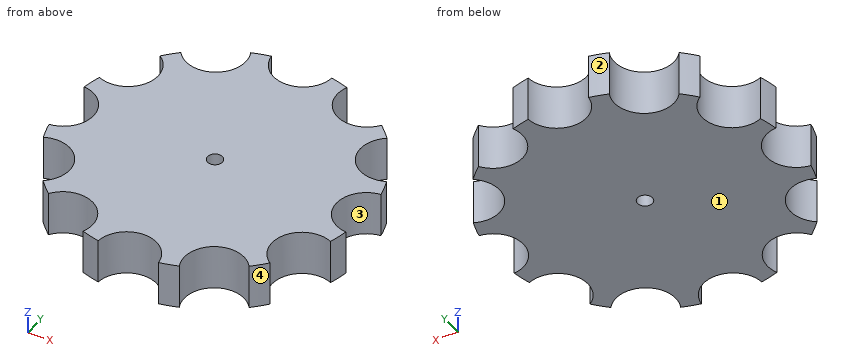
```python
from build123d import *

# Parameters (mm, degrees)
BOSS_EXTRUDE3_DEPTH = 15
SKETCH3_R           = 2.5
CUT_EXTRUDE2_DEPTH  = 15


with BuildPart() as part:
    # Sketch1 → Boss-Extrude3 (new body)
    with BuildSketch(Plane.XY):
        with BuildLine():
            ThreePointArc((48.999319531, 9.953224878), (48.296291314, 12.940952255), (47.411267921, 15.879914172))
            ThreePointArc((47.411267921, 15.879914172), (34.638070137, 19.998299118), (37.458043043, 33.119405359))
            ThreePointArc((37.458043043, 33.119405359), (35.355339059, 35.355339059), (33.119405359, 37.458043043))
            ThreePointArc((33.119405359, 37.458043043), (19.998299118, 34.638070137), (15.879914172, 47.411267921))
            ThreePointArc((15.879914172, 47.411267921), (12.940952255, 48.296291314), (9.953224878, 48.999319531))
            ThreePointArc((9.953224878, 48.999319531), (0, 39.996598235), (-9.953224878, 48.999319531))
            ThreePointArc((-9.953224878, 48.999319531), (-12.940952255, 48.296291314), (-15.879914172, 47.411267921))
            ThreePointArc((-15.879914172, 47.411267921), (-19.998299118, 34.638070137), (-33.119405359, 37.458043043))
            ThreePointArc((-33.119405359, 37.458043043), (-35.355339059, 35.355339059), (-37.458043043, 33.119405359))
            ThreePointArc((-37.458043043, 33.119405359), (-34.638070137, 19.998299118), (-47.411267921, 15.879914172))
            ThreePointArc((-47.411267921, 15.879914172), (-48.296291314, 12.940952255), (-48.999319531, 9.953224878))
            ThreePointArc((-48.999319531, 9.953224878), (-39.996598235, 0), (-48.999319531, -9.953224878))
            ThreePointArc((-48.999319531, -9.953224878), (-48.296291314, -12.940952255), (-47.411267921, -15.879914172))
            ThreePointArc((-47.411267921, -15.879914172), (-34.638070137, -19.998299118), (-37.458043043, -33.119405359))
            ThreePointArc((-37.458043043, -33.119405359), (-35.355339059, -35.355339059), (-33.119405359, -37.458043043))
            ThreePointArc((-33.119405359, -37.458043043), (-19.998299118, -34.638070137), (-15.879914172, -47.411267921))
            ThreePointArc((-15.879914172, -47.411267921), (-12.940952255, -48.296291314), (-9.953224878, -48.999319531))
            ThreePointArc((-9.953224878, -48.999319531), (0, -39.996598235), (9.953224878, -48.999319531))
            ThreePointArc((9.953224878, -48.999319531), (12.940952255, -48.296291314), (15.879914172, -47.411267921))
            ThreePointArc((15.879914172, -47.411267921), (19.998299118, -34.638070137), (33.119405359, -37.458043043))
            ThreePointArc((33.119405359, -37.458043043), (35.355339059, -35.355339059), (37.458043043, -33.119405359))
            ThreePointArc((37.458043043, -33.119405359), (34.638070137, -19.998299118), (47.411267921, -15.879914172))
            ThreePointArc((47.411267921, -15.879914172), (48.296291314, -12.940952255), (48.999319531, -9.953224878))
            ThreePointArc((48.999319531, -9.953224878), (39.996598235, 0), (48.999319531, 9.953224878))
        make_face()
    extrude(amount=BOSS_EXTRUDE3_DEPTH)

    # Sketch3 → Cut-Extrude2 (cut)
    with BuildSketch(Plane(origin=(0, 0, 0), x_dir=(-1, 0, 0), z_dir=(0, 0, -1))):
        Circle(SKETCH3_R)
    extrude(amount=-CUT_EXTRUDE2_DEPTH, mode=Mode.SUBTRACT)


solid = part.part
```
Input: part model. Units: mm. Frame: model coordinates. Face numbers are marked on the shaded views. Coordinates: 2 decimals unless noted, no trailing zeros. Write each loop counter-clockwise with the first axis right and the second up, starting at its lowest first coordinate (ties: lowest second). Pieces come first, ordered by that corner, then holes. Notation, with made-up numbers: M 67,4.5 L 90,4.5 A18 cw 90,17.5 Z; hole C 70.25,-37 d5. An arc over 180 degrees is marked long. Use one line per item in the form item = value.
Q1. Section C-C (z = 10.5). Return loops of the section in (x, y), plus the area to 3 significant figures.
Answer below:
outline = M -49,-9.95 A50 ccw -47.41,-15.88 A10 cw -37.46,-33.12 A50 ccw -33.12,-37.46 A10 cw -15.88,-47.41 A50 ccw -9.95,-49 A10 cw 9.95,-49 A50 ccw 15.88,-47.41 A10 cw 33.12,-37.46 A50 ccw 37.46,-33.12 A10 cw 47.41,-15.88 A50 ccw 49,-9.95 A10 cw 49,9.95 A50 ccw 47.41,15.88 A10 cw 37.46,33.12 A50 ccw 33.12,37.46 A10 cw 15.88,47.41 A50 ccw 9.95,49 A10 cw -9.95,49 A50 ccw -15.88,47.41 A10 cw -33.12,37.46 A50 ccw -37.46,33.12 A10 cw -47.41,15.88 A50 ccw -49,9.95 A10 cw Z; hole C 0,0 d5
area = 6,030 mm²
Q2. Material intervals for probe 1 along Y at (x, z) = (0, 3.75); probe 2 along X at (y, z) = (-43, 14.5); probe 3 along Y at (x, z) = (37.5, 4.5), sorted ascending. Write a range as from..to.
Answer below:
probe_1 = -40..-2.5, 2.5..40
probe_2 = -15..-7.15, 7.15..15
probe_3 = -16.85..16.85
Q3. First-contact query: pin 1 (4 mm diameter, centred on x = 7, z = 2.5, fed in from +Y); pin 2 (4 mm diameter, centred on x = 0, y = 0, fed in from -Z); pin 3 (5 mm diameter, centred on y = -29, z = 5.5, fed in from +X); pin 4 (4 mm diameter, centred on x = 17, z = 7, fed in from +Y). Flat tips, straight axial feed; report the tip coordinate or a pass-through.
Answer below:
pin_1 = 45.63
pin_2 = through
pin_3 = 35.7
pin_4 = 47.7
Q4. Section D-D (y = 31.5). Return loops of the section in (x, z), plus the area to 3 significant figures.
Answer below:
outline = M -35.7,0 L 35.7,0 L 35.7,15 L -35.7,15 Z
area = 1,070 mm²
Q5. Draft query along Y for the marked faces 1, 2, 3 and 4. Return one class per face: released by +Y, released by -Y, zero draft, split by the parting line, or undercut.
Answer below:
face_1 = zero draft
face_2 = released by +Y
face_3 = undercut
face_4 = released by -Y
Q6. Section A-A (y = 0). Return loops of the section in (x, z).
Answer below:
outline = M -40,0 L -2.5,0 L -2.5,15 L -40,15 Z; M 2.5,0 L 40,0 L 40,15 L 2.5,15 Z
